Design review of the part built by this model. Coordinates are the model's own, in mm. Coordinates: 2 decimals unless noted, no trailing zeros. Write each loop counter-clockwise with the first axis right and the second up, starting at its lowest first coordinate (ties: lowest second). Pieces come first, ordered by that corner, then holes. Notation, with made-up numbers: (73, 36.25) - (121, 36.25) arc R19 ccw to (121, 55.25) - close; hole circle Ø4 at (-14.75, 44). An arc over 180 degrees is marked (long way). One line per item, written item: value.
from build123d import *

# Parameters (mm, degrees)
SKETCH1_R           = 3.96875
BOSS_EXTRUDE1_DEPTH = 31.475
SKETCH3_R           = 1.25
CUT_EXTRUDE1_DEPTH  = 4.5
SKETCH4_R           = 1.352058412
CUT_EXTRUDE2_DEPTH  = 4.5
CHAMFER1_SIZE       = 0.5


with BuildPart() as part:
    # Sketch1 → Boss-Extrude1 (new body)
    with BuildSketch(Plane.XY):
        Circle(SKETCH1_R)
    extrude(amount=BOSS_EXTRUDE1_DEPTH)

    # Sketch3 → Cut-Extrude1 (cut)
    with BuildSketch(Plane.XY.offset(31.475)):
        Circle(SKETCH3_R)
    extrude(amount=-CUT_EXTRUDE1_DEPTH, mode=Mode.SUBTRACT)

    # Sketch4 → Cut-Extrude2 (cut)
    with BuildSketch(Plane(origin=(0, 0, 0), x_dir=(-1, 0, 0), z_dir=(0, 0, -1))):
        Circle(SKETCH4_R)
    extrude(amount=-CUT_EXTRUDE2_DEPTH, mode=Mode.SUBTRACT)

    # Chamfer1
    chamfer1_edges = [part.edges().sort_by_distance(p)[0] for p in [
        (1.352058412, 0, 0),
        (-3.96875, 0, 0),
        (-3.96875, 0, 31.475),
        (-1.25, 0, 31.475),
    ]]
    chamfer(chamfer1_edges, length=CHAMFER1_SIZE)


solid = part.part
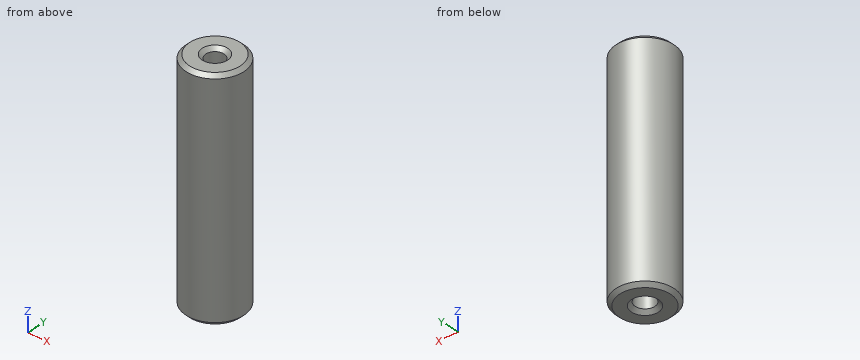
1. Wall thickness on line 1 along Y through (x, z) = (0, 2.6); line 2 along Y through (x, z) = (0, 28.6); line 3 along Z through (x, y) = (-1.75, -3): over which ranges is each line inside the solid? List them lowest first.
Answer block:
line 1: y = -3.97 to -1.35, 1.35 to 3.97
line 2: y = -3.97 to -1.25, 1.25 to 3.97
line 3: z = 0 to 31.47
2. Consider section C-C, the plane z = 20. Write out the cut boundary in (x, y), then the cut area to 3 significant figures.
Answer block:
outline: circle Ø7.94 at (0, 0)
area: 49.5 mm^2
3. Insertion check: pin 1 Ø3 at (x, z) = (0.5, 7) entering from +Y; pin 2 Ø1 at (y, z) = (-3, 5) entering from -X; pin 3 Ø2 at (x, y) = (0, 0) entering from -Z. Each pin has a flat end and moves straight along its axis. Give the tip position at first contact, or say it passes through.
Answer block:
pin 1: stops at y = 3.97
pin 2: stops at x = -3.08
pin 3: stops at z = 4.5
4. Consider section A-A, the plane x = 0. Write out the cut boundary in (y, z) (3 decimals), then the cut area to 3 significant figures.
Answer block:
outline: (-3.969, 0.5) - (-3.469, 0) - (-1.852, 0) - (-1.352, 0.5) - (-1.352, 4.5) - (1.352, 4.5) - (1.352, 0.5) - (1.852, 0) - (3.469, 0) - (3.969, 0.5) - (3.969, 30.975) - (3.469, 31.475) - (1.75, 31.475) - (1.25, 30.975) - (1.25, 26.975) - (-1.25, 26.975) - (-1.25, 30.975) - (-1.75, 31.475) - (-3.469, 31.475) - (-3.969, 30.975) - close
area: 225 mm^2
